from build123d import *

# Parameters (mm, degrees)
BOSS_EXTRU_1_DEPTH      = 54.4
ESQUISSE2_R             = 6.2
ENL_V_MAT_EXTRU_1_DEPTH = 55.4
BOSS_EXTRU_2_DEPTH      = 54.4
ESQUISSE4_R             = 3.5
BOSS_EXTRU_3_DEPTH      = 2.6
ESQUISSE5_R             = 5.1
BOSS_EXTRU_4_DEPTH      = 3


with BuildPart() as part:
    # Esquisse1 → Boss.-Extru.1 (new body)
    with BuildSketch(Plane(origin=(0, 0, 0), x_dir=(1, 0, 0), z_dir=(0, 1, 0))):
        with BuildLine():
            ThreePointArc((-33.897137082, 23.942307692), (-41.5, 0), (-33.897137082, -23.942307692))
            ThreePointArc((-33.897137082, -23.942307692), (-30.41283318, -24.54199621), (-29.813144663, -21.057692308))
            ThreePointArc((-29.813144663, -21.057692308), (-36.5, 0), (-29.813144663, 21.057692308))
            ThreePointArc((-29.813144663, 21.057692308), (-30.41283318, 24.54199621), (-33.897137082, 23.942307692))
        make_face()
    extrude(amount=BOSS_EXTRU_1_DEPTH)

    # Esquisse2 → Enlèv. mat.-Extru.1 (cut, through all)
    with BuildSketch(Plane(origin=(0, 54.4, 0), x_dir=(1, 0, 0), z_dir=(0, 1, 0))):
        with Locations((-39.130938787, 15)):
            Circle(ESQUISSE2_R)
        with Locations((-39.130938787, -15)):
            Circle(ESQUISSE2_R)
    extrude(amount=-ENL_V_MAT_EXTRU_1_DEPTH, mode=Mode.SUBTRACT)

    # Esquisse3 → Boss.-Extru.2 (add)
    with BuildSketch(Plane.XZ):
        with BuildLine():
            Line((-47.130938787, 15), (-47.130938787, -15))
            ThreePointArc((-47.130938787, -15), (-45.439748727, -19.919239489), (-41.081209501, -22.758636745))
            Line((-41.081209501, -22.758636745), (-32.46460047, -24.924573983))
            ThreePointArc((-32.46460047, -24.924573983), (-29.793288851, -23.913777296), (-29.813144663, -21.057692308))
            ThreePointArc((-29.813144663, -21.057692308), (-31.505533615, -18.429632433), (-32.966857258, -15.666407455))
            ThreePointArc((-32.966857258, -15.666407455), (-44.920174268, -17.219178351), (-34.991734648, -10.384050575))
            ThreePointArc((-34.991734648, -10.384050575), (-36.5, 0), (-34.991734648, 10.384050575))
            ThreePointArc((-34.991734648, 10.384050575), (-44.920174268, 17.219178351), (-32.966857258, 15.666407455))
            ThreePointArc((-32.966857258, 15.666407455), (-31.505533615, 18.429632433), (-29.813144663, 21.057692308))
            ThreePointArc((-29.813144663, 21.057692308), (-29.793288851, 23.913777296), (-32.46460047, 24.924573983))
            Line((-32.46460047, 24.924573983), (-41.081209501, 22.758636745))
            ThreePointArc((-41.081209501, 22.758636745), (-45.439748727, 19.919239489), (-47.130938787, 15))
        make_face()
    extrude(amount=-BOSS_EXTRU_2_DEPTH)

    # Esquisse4 → Boss.-Extru.3 (add)
    with BuildSketch(Plane.XZ):
        with BuildLine():
            Line((-47.130938787, 15), (-47.130938787, -15))
            ThreePointArc((-47.130938787, -15), (-45.439748727, -19.919239489), (-41.081209501, -22.758636745))
            Line((-41.081209501, -22.758636745), (-32.46460047, -24.924573983))
            ThreePointArc((-32.46460047, -24.924573983), (-29.793288851, -23.913777296), (-29.813144663, -21.057692308))
            ThreePointArc((-29.813144663, -21.057692308), (-36.5, 0), (-29.813144663, 21.057692308))
            ThreePointArc((-29.813144663, 21.057692308), (-29.793288851, 23.913777296), (-32.46460047, 24.924573983))
            Line((-32.46460047, 24.924573983), (-41.081209501, 22.758636745))
            ThreePointArc((-41.081209501, 22.758636745), (-45.439748727, 19.919239489), (-47.130938787, 15))
        make_face()
        with Locations((-39.130938787, 15)):
            Circle(ESQUISSE4_R, mode=Mode.SUBTRACT)
        with Locations((-39.130938787, -15)):
            Circle(ESQUISSE4_R, mode=Mode.SUBTRACT)
    extrude(amount=BOSS_EXTRU_3_DEPTH)

    # Esquisse5 → Boss.-Extru.4 (add)
    with BuildSketch(Plane.XZ.offset(2.6)):
        with BuildLine():
            Line((-32.46460047, 24.924573983), (-41.081209501, 22.758636745))
            ThreePointArc((-41.081209501, 22.758636745), (-45.439748727, 19.919239489), (-47.130938787, 15))
            Line((-47.130938787, 15), (-47.130938787, -15))
            ThreePointArc((-47.130938787, -15), (-45.439748727, -19.919239489), (-41.081209501, -22.758636745))
            Line((-41.081209501, -22.758636745), (-32.46460047, -24.924573983))
            ThreePointArc((-32.46460047, -24.924573983), (-29.793288851, -23.913777296), (-29.813144663, -21.057692308))
            ThreePointArc((-29.813144663, -21.057692308), (-36.5, 0), (-29.813144663, 21.057692308))
            ThreePointArc((-29.813144663, 21.057692308), (-29.793288851, 23.913777296), (-32.46460047, 24.924573983))
        make_face()
        with Locations((-39.130938787, 15)):
            Circle(ESQUISSE5_R, mode=Mode.SUBTRACT)
        with Locations((-39.130938787, -15)):
            Circle(ESQUISSE5_R, mode=Mode.SUBTRACT)
    extrude(amount=BOSS_EXTRU_4_DEPTH)


solid = part.part
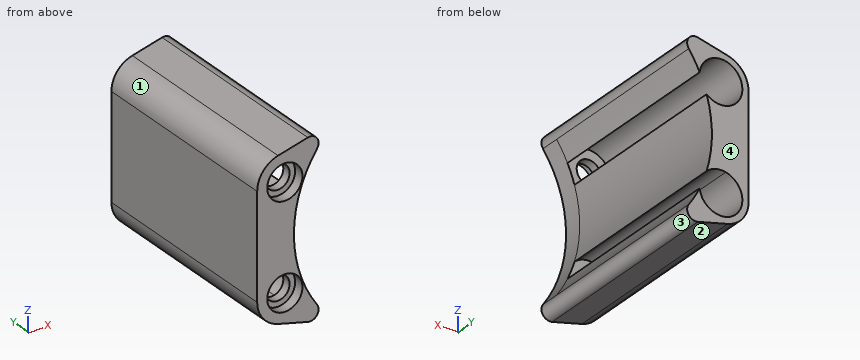
Verification items for the finished model (mm, model axes). Face numbers are marked on the shaded views. Round coordinates to 2 decimals unless told otherwise and drop trailing zeros. Loops run counter-clockwise (first coordinate to the right, second up) from the corner with the lowest first, then second, coordinate; pieces in that order, holes last. Notation, with made-up numbers: (-10.75, -16.75) - (46.25, -16.75) arc R8 ccw to (46.25, -12.75) - close; hole circle Ø1 at (44, 43). An arc over 180 degrees is marked (long way). Write item = value, one per line.
Q1. Material ranges on L1, parallel to Z at x = -39.25, y = -2; L2, parallel to Z at x = -36.75, y = 41.5; L3, parallel to Z at x = -29.75, y = 6, recorded low to high.
Here are the results:
L1 = -23.22 to -18.5, -11.5 to 11.5, 18.5 to 23.22
L2 = -23.85 to -20.72, -9.28 to 9.28, 20.72 to 23.85
L3 = -23.85 to -21.15, 21.15 to 23.85
Q2. Sectioned sample at A-A on z = -14. Record the boundary of the cut face in (x, y).
Here are the results:
outline = (-47.13, -5.6) - (-44.13, -5.6) - (-44.13, -2.6) - (-42.49, -2.6) - (-42.49, 0) - (-45.25, 0) - (-45.25, 54.4) - (-47.13, 54.4) - close; (-35.78, -2.6) - (-34.13, -2.6) - (-34.13, -5.6) - (-33.71, -5.6) - (-33.71, 0) - (-35.78, 0) - close
Q3. Sectioned sample at C-C on x = -37.5. Record the boundary of the cut face in (y, z), plus the area to 3 significant figures.
Here are the results:
outline = (-5.6, -23.66) - (54.4, -23.66) - (54.4, -20.98) - (0, -20.98) - (0, -18.1) - (-2.6, -18.1) - (-2.6, -19.83) - (-5.6, -19.83) - close; (-5.6, -10.17) - (-2.6, -10.17) - (-2.6, -11.9) - (0, -11.9) - (0, -9.02) - (54.4, -9.02) - (54.4, 9.02) - (0, 9.02) - (0, 11.9) - (-2.6, 11.9) - (-2.6, 10.17) - (-5.6, 10.17) - close; (-5.6, 19.83) - (-2.6, 19.83) - (-2.6, 18.1) - (0, 18.1) - (0, 20.98) - (54.4, 20.98) - (54.4, 23.66) - (-5.6, 23.66) - close
area = 1,450 mm^2
Q4. Depth check by flat-ended pin: pin 1 (8 mm diameter, centred on x = -39.13, z = -15, fed in from +Y); pin 2 (9 mm diameter, centred on x = -39.13, z = -15, fed in from -Y); pin 3 (1 mm diameter, centred on x = -36, y = 43.5, fed in from +Z). Enter the tip coordinate at first touch or a pass-through.
Here are the results:
pin_1 = 0
pin_2 = -2.6
pin_3 = 24.16
Q5. Sectioned sample at D-D on z = -4.5. Record the boundary of the cut face in (x, y).
Here are the results:
outline = (-47.13, -5.6) - (-36.22, -5.6) - (-36.22, 54.4) - (-47.13, 54.4) - close
Q6. Sectioned sample at B-B on y = 47. Record the boundary of the cut face in (x, z).
Here are the results:
outline = (-47.13, -15) arc R8 ccw to (-41.08, -22.76) - (-32.46, -24.92) arc R2.5 ccw to (-29.81, -21.06) arc R36.5 cw to (-32.97, -15.67) arc R6.2 cw (long way) to (-34.99, -10.38) arc R36.5 cw to (-34.99, 10.38) arc R6.2 cw (long way) to (-32.97, 15.67) arc R36.5 cw to (-29.81, 21.06) arc R2.5 ccw to (-32.46, 24.92) - (-41.08, 22.76) arc R8 ccw to (-47.13, 15) - close
Q7. Mould release check, pull along Z, two halves, no side actions. Record for the marked faces 1, 2, 3 and 4: +Z half, -Z half, draft (parallel to the pull), parting line (faces both ways), or undercut.
Here are the results:
face_1 = +Z half
face_2 = -Z half
face_3 = undercut
face_4 = draft
